from build123d import *

# Parameters (mm, degrees)
F1_DEPTH = 50
F3_DEPTH = 55


with BuildPart() as f1:
    # F0 (on Top) → F1 (new body)
    with BuildSketch(Plane.XY):
        Polygon((6.523423, 65.423498), (-20.813363, 62.254017), (-44.497616, 48.239678), (-60.434112, 25.80369), (-65.867287, -1.174563), (-59.857696, -28.030294), (-43.444451, -50.119905), (-19.465552, -63.6239), (7.932832, -66.207316), (34.013272, -57.423458), (54.266222, -38.791133), (65.189763, -13.532041), (64.895117, 13.986292), (53.433229, 39.005697), (32.785965, 57.200091), align=None)
    extrude(amount=F1_DEPTH)

    # F2 (on face) → F3 (cut)
    with BuildSketch(Plane(origin=(0, 0, 0), x_dir=(1, 0, 0), z_dir=(0, 0, -1))):
        Polygon((64.895117, -13.986292), (0, 0), (6.523423, -65.423498), (32.785965, -57.200091), (53.433229, -39.005697), align=None)
    extrude(amount=-F3_DEPTH, mode=Mode.SUBTRACT)


solid = f1.part
The listing builds one solid part. Answer for the finished solid, in the listing's coordinates (mm). Give positions to 0.01 mm unless a question says otherwise; leave off trailing zeros. Loops run counter-clockwise (first coordinate to the right, second up) from the corner with the lowest first, then second, coordinate; pieces in that order, holes last. Notation, with made-up numbers: (72.25, -16.75) - (128.25, -16.75) arc R19 cw to (128.25, 11.25) - close; hole circle Ø2 at (83.5, 83). An arc over 180 degrees is marked (long way). Answer as a JSON object with one key per item and string values.
1. A cutting plane is placed at C-C (z = 13). Write down the section's boundary in (x, y).
Determined:
{"outline": "(-65.87, -1.17) - (-59.86, -28.03) - (-43.44, -50.12) - (-19.47, -63.62) - (7.93, -66.21) - (34.01, -57.42) - (54.27, -38.79) - (65.19, -13.53) - (64.9, 13.99) - (0, 0) - (6.52, 65.42) - (-20.81, 62.25) - (-44.5, 48.24) - (-60.43, 25.8) - close"}
2. Flat-ended cylindrical pins translate along their axes: pin 1 Ø1 at (y, z) = (-28.5, 22.5) entering from -X; pin 2 Ø4 at (x, z) = (-21.5, 17.5) entering from +Y; pin 3 Ø10 at (y, z) = (15.5, 8) entering from +X. Find the tip coordinate at first contact, or state that the pin passes through.
Determined:
{"pin 1": "x = -59.86", "pin 2": "y = 62.41", "pin 3": "x = 64.93"}
3. Find the intervals of material crossed by L1, parallel to Y at x = 15.5, z = 19; L2, parallel to Y at x = 38.5, z = 19; L3, parallel to X at y = 31, z = 14, in increasing order. Write a range as [from, to].
Determined:
{"L1": "[-63.66, 3.34]", "L2": "[-53.3, 8.3]", "L3": "[-56.74, 3.09]"}
4. A cutting plane is placed at D-D (y = -45.5). Write down the section's boundary in (x, z).
Determined:
{"outline": "(-46.88, 0) - (46.97, 0) - (46.97, 50) - (-46.88, 50) - close"}
5. A cutting plane is placed at A-A (y = 5). Write down the section's boundary in (x, z).
Determined:
{"outline": "(-64.62, 0) - (0.5, 0) - (0.5, 50) - (-64.62, 50) - close; (23.2, 0) - (64.99, 0) - (64.99, 50) - (23.2, 50) - close"}
6. For a pull along X with two mould halves and no side action, classify faces 1 (the flat face through (43.998, -48.238, 24.65)), 2 (the flat face through (-52.354, 37.179, 24.65)), 3 (the flat face through (3.216, 32.254, 24.65)), 4 (the flat face through (-1, -14, 50)) as pulls with the +X half, pulls with the -X half, needs draft (parallel to the pull), parting line crosses it, or undercut.
Determined:
{"face 1": "pulls with the +X half", "face 2": "pulls with the -X half", "face 3": "undercut", "face 4": "needs draft"}
7. A cutting plane is placed at B-B (x = 4.5). Write down the section's boundary in (y, z).
Determined:
{"outline": "(-65.88, 0) - (0.97, 0) - (0.97, 50) - (-65.88, 50) - close; (45.13, 0) - (65.19, 0) - (65.19, 50) - (45.13, 50) - close"}
